from build123d import *

# Parameters (mm, degrees)
SKETCH_1_R      = 0.5
EXTRUDE_1_DEPTH = 1
EXTRUDE_START   = -2.45
EXTRUDE_2_DEPTH = 2.45
FILLET_1_R      = 0.2


with BuildPart() as part:
    # 草图1 → 凸台-拉伸1 (new body)
    with BuildSketch(Plane.XY):
        with BuildLine():
            Line((-14.016792693, -2.096749739), (-6.313489141, -2.525837459))
            ThreePointArc((-6.313489141, -2.525837459), (-6.8, 0), (-6.313489141, 2.525837459))
            Line((-6.313489141, 2.525837459), (-14.016792693, 2.096749739))
            ThreePointArc((-14.016792693, 2.096749739), (-16, 0), (-14.016792693, -2.096749739))
        make_face()
        with Locations((-10.3, 0)):
            Circle(SKETCH_1_R, mode=Mode.SUBTRACT)
        with Locations((-8.3, 0)):
            Circle(SKETCH_1_R, mode=Mode.SUBTRACT)
        with Locations((-12.3, 0)):
            Circle(SKETCH_1_R, mode=Mode.SUBTRACT)
    extrude(amount=EXTRUDE_1_DEPTH)

    # 草图3 → 凸台-拉伸2 (add)
    with BuildSketch(Plane.XY.offset(1).offset(EXTRUDE_START)):
        with BuildLine():
            Line((-6.313489141, 4.028162673), (-14.100216045, 3.594428124))
            ThreePointArc((-14.100216045, 3.594428124), (-17.5, 0), (-14.100216045, -3.594428124))
            Line((-14.100216045, -3.594428124), (-6.313489141, -4.028162673))
            Line((-6.313489141, -4.028162673), (-6.313489141, -2.525837459))
            Line((-6.313489141, -2.525837459), (-14.016792693, -2.096749739))
            ThreePointArc((-14.016792693, -2.096749739), (-16, 0), (-14.016792693, 2.096749739))
            Line((-14.016792693, 2.096749739), (-6.313489141, 2.525837459))
            Line((-6.313489141, 2.525837459), (-6.313489141, 4.028162673))
        make_face()
    extrude(amount=EXTRUDE_2_DEPTH)

    # 圆角1
    fillet_1_edges = [part.edges().sort_by_distance(p)[0] for p in [
        (-10.206852593, 3.811295398, 1),
        (-17.5, 0, 1),
        (-10.206852593, -3.811295398, 1),
        (-17.5, 0, -1.45),
        (-10.206852593, -3.811295398, -1.45),
        (-6.313489141, -4.028162673, -0.225),
        (-6.313489141, 4.028162673, -0.225),
        (-10.206852593, 3.811295398, -1.45),
    ]]
    fillet(fillet_1_edges, radius=FILLET_1_R)


solid = part.part
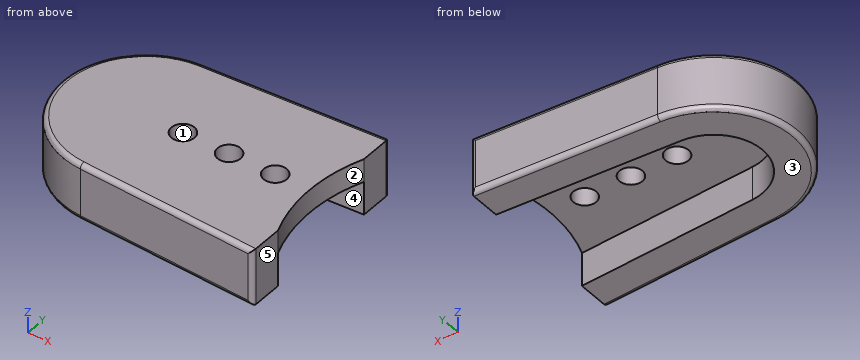
Verification items for the finished model (mm, model axes). Face numbers are marked on the shaded views. A direction names the side the tool comes from. Give positions to 0.01 mm unless a question says otherwise; leave off trailing zeros. Loops run counter-clockwise (first coordinate to the right, second up) from the corner with the lowest first, then second, coordinate; pieces in that order, holes last.
1) Sectioned sample at A-A, the plane z = 0.2. Enter the section's corners in (x, y).
2) Depth check by flat-ended pin: pin 1 Ø1.5 at (x, y) = (-9, -0.5) entering from -Z. Enter the tip coordinate at first touch or a pass-through.
3) Draft check along X on the marked faces 1, 2 and 3. Enter one of: pulls with the +X half, pulls with the -X half, needs draft (parallel to the pull), parting line crosses it, or undercut.
4) Thickness scan on line 1 along Z through (x, y) = (-7.5, -1); line 2 along Y through (x, z) = (-8.25, -0.25); line 3 along Y through (x, z) = (-14.75, -1). Record the ranges inside material, lowest first.
5) Sectioned sample at B-B, the plane y = 0. Enter the section's corners in (x, z).
6) Set-up check for the marked faces 4 and 5: record each of +Z, -Z, +X, -X, +Y, -Y from which the full face is reachable in a straight line by a thin tool's end or side.
Answers:
1. outline: (-14.1, -3.59) - (-6.52, -4.02) arc R0.2 ccw to (-6.31, -3.82) - (-6.31, -2.53) arc R6.8 cw to (-6.31, 2.53) - (-6.31, 3.82) arc R0.2 ccw to (-6.52, 4.02) - (-14.1, 3.59) arc R3.6 ccw to start; hole circle Ø1 at (-12.3, 0); hole circle Ø1 at (-10.3, 0); hole circle Ø1 at (-8.3, 0)
2. pin 1: stops at z = 0
3. face 1: undercut
3. face 2: pulls with the +X half
3. face 3: needs draft
4. line 1: z = 0 to 1
4. line 2: y = -3.92 to -2.42, 2.42 to 3.92
4. line 3: y = -3.5 to -1.92, 1.92 to 3.5
5. outline: (-17.5, -1.25) arc R0.2 ccw to (-17.3, -1.45) - (-16, -1.45) - (-16, 0) - (-12.8, 0) - (-12.8, 1) - (-17.3, 1) arc R0.2 ccw to (-17.5, 0.8) - close; (-11.8, 0) - (-10.8, 0) - (-10.8, 1) - (-11.8, 1) - close; (-9.8, 0) - (-8.8, 0) - (-8.8, 1) - (-9.8, 1) - close; (-7.8, 0) - (-6.8, 0) - (-6.8, 1) - (-7.8, 1) - close
6. face 4: -Z, +X
6. face 5: +Z, -Z, +X, +Y, -Y
